```python
from build123d import *

# Parameters (mm, degrees)
F0_W     = 42
F0_H     = 5.7
F1_DEPTH = 5.8


with BuildPart() as f1:
    # F0 (on Top) → F1 (new body)
    with BuildSketch(Plane.XY):
        Polygon((87.5, 53.65), (87.5, 70), (-87.5, 70), (-87.5, 53.65), (-93.85, 53.65), (-93.85, 11.35), (-87.5, 11.35), (-87.5, -8.175), (-93.85, -8.175), (-93.85, -50.475), (-87.5, -50.475), (-87.5, -70), (87.5, -70), (87.5, -50.475), (93.85, -50.475), (93.85, -8.175), (87.5, -8.175), (87.5, 11.35), (93.85, 11.35), (93.85, 53.65), align=None)
        with BuildLine():
            ThreePointArc((-44.294584, -48.020755), (-44.821792, -49.293547), (-46.094584, -49.820755))
            Line((-46.094584, -49.820755), (-60.533295, -49.820757))
            ThreePointArc((-60.533295, -49.820757), (-61.806087, -49.293549), (-62.333295, -48.020757))
            Line((-62.333295, -48.020757), (-62.333295, -28.613132))
            ThreePointArc((-62.333295, -28.613132), (-61.806087, -27.34034), (-60.533295, -26.813132))
            Line((-60.533295, -26.813132), (-46.094584, -26.813134))
            ThreePointArc((-46.094584, -26.813134), (-44.821792, -27.340342), (-44.294584, -28.613134))
            Line((-44.294584, -28.613134), (-44.294584, -34.793572))
            Line((-44.294584, -34.793572), (-48.72147, -34.793572))
            Line((-48.72147, -34.793572), (-48.72147, -30.456954))
            Line((-48.72147, -30.456954), (-57.906409, -30.456954))
            Line((-57.906409, -30.456954), (-57.906409, -46.176934))
            Line((-57.906409, -46.176934), (-48.72147, -46.176934))
            Line((-48.72147, -46.176934), (-48.72147, -41.569373))
            Line((-48.72147, -41.569373), (-44.294584, -41.569373))
            Line((-44.294584, -41.569373), (-44.294584, -48.020755))
        make_face(mode=Mode.SUBTRACT)
        Polygon((-37.007503, -49.820755), (-41.524656, -49.76053), (-33.755004, -26.813132), (-29.057175, -26.813132), (-21.287593, -49.76053), (-25.834929, -49.820755), (-31.436272, -31.842268), align=None, mode=Mode.SUBTRACT)
        Polygon((-59.096379, -24.434737), (-62.305008, -24.434737), (-62.305008, -13.392651), (-58.836246, -13.392651), (-56.350317, -19.318423), (-53.936685, -13.392651), (-50.496843, -13.392651), (-50.496843, -24.434737), (-53.662093, -24.434737), (-53.662093, -19.506257), (-55.064043, -23.957851), (-57.694499, -23.957851), (-59.096379, -19.506257), align=None, mode=Mode.SUBTRACT)
        Polygon((-45.771218, -20.069901), (-45.771218, -24.434737), (-49.037616, -24.434737), (-49.037616, -13.392651), (-40.134498, -13.392651), (-40.134498, -16.051955), (-45.771218, -16.051955), (-45.771218, -17.555053), (-41.406382, -17.555053), (-41.406382, -20.069901), align=None, mode=Mode.SUBTRACT)
        Polygon((-37.605611, -24.434737), (-40.929777, -24.405818), (-37.114195, -13.392651), (-33.631044, -13.392651), (-29.815392, -24.405818), (-33.168477, -24.434737), (-35.379814, -16.919111), align=None, mode=Mode.SUBTRACT)
        with Locations((-41.5, 25.8)):
            Rectangle(F0_W, F0_H, mode=Mode.SUBTRACT)
        with Locations((-41.5, 62.15)):
            Rectangle(F0_W, F0_H, mode=Mode.SUBTRACT)
        with Locations((41.5, 25.8)):
            Rectangle(F0_W, F0_H, mode=Mode.SUBTRACT)
        with Locations((41.5, 62.15)):
            Rectangle(F0_W, F0_H, mode=Mode.SUBTRACT)
    extrude(amount=F1_DEPTH)


solid = f1.part
```
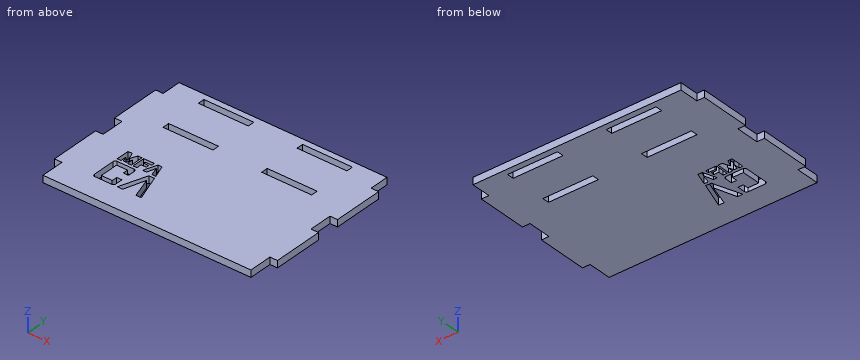
Source: CAD feature listing. Evaluate the final solid. Frame: model axes, mm. Round coordinates to 2 decimals unless told otherwise and drop trailing zeros. Write each loop counter-clockwise with the first axis right and the second up, starting at its lowest first coordinate (ties: lowest second). Pieces come first, ordered by that corner, then holes. Notation, with made-up numbers: M 25.5,-17 L 70.5,-17 A11 ccw 70.5,-6 Z; hole C 7,33.5 d8. An arc over 180 degrees is marked long. Answer as a JSON object with one key per item and string values. Group by question number.
(1) Ray query, line 1 (X direction, y = 25, z = 5); line 2 (Y direction, x = 55, z = 2.5); line 3 (X direction, y = -17.5, z = 3.5) (3 decimals). Return the intervals inside material, ascending. Write a range as [from, to].
(2) Section query A-A on x = 57.5. Output: boundary loops of the cut face in (y, z), then the cut area to 3 significant figures.
(3) First-contact query: pin 1 (3 mm diameter, centred on x = 89.5, z = 3.5, fed in from -Y) (3 decimals). Flat tip, straight axial feed; report the tip coordinate or a pass-through.
(4) Section query B-B on z = 2.65. State how many separate pieces and enclosed holes the cut face has, then the cut area to 3 significant figures.
Computed values:
{
 "1": {"line 1": "[-93.85, -62.5], [-20.5, 20.5], [62.5, 93.85]", "line 2": "[-70, 22.95], [28.65, 59.3], [65, 70]", "line 3": "[-93.85, -62.305], [-57.113, -55.61], [-50.497, -49.038], [-45.771, -38.537], [-35.552, -35.209], [-32.208, 93.85]"},
 "2": {"outline": "M -70,0 L 22.95,0 L 22.95,5.8 L -70,5.8 Z; M 28.65,0 L 59.3,0 L 59.3,5.8 L 28.65,5.8 Z; M 65,0 L 70,0 L 70,5.8 L 65,5.8 Z", "area": "746 mm^2"},
 "3": {"pin 1": "y = -50.475"},
 "4": {"separate pieces": "1", "enclosed holes": "9", "area": "24,000 mm^2"}
}
